from build123d import *

# Parameters (mm, degrees)
SALIENTE_EXTRUIR1_DEPTH = 2.5
CROQUIS2_R              = 3.175
CORTAR_EXTRUIR1_DEPTH   = 86.532786696


with BuildPart() as part:
    # Croquis1 → Saliente-Extruir1 (new, symmetric)
    with BuildSketch(Plane.XY):
        with BuildLine():
            Line((-85.24, 5), (85.24, 5))
            Line((85.24, 5), (85.24, -1))
            ThreePointArc((85.24, -1), (84.068427125, -3.828427125), (81.24, -5))
            Line((81.24, -5), (-81.24, -5))
            ThreePointArc((-81.24, -5), (-84.068427125, -3.828427125), (-85.24, -1))
            Line((-85.24, -1), (-85.24, 5))
        make_face()
    extrude(amount=SALIENTE_EXTRUIR1_DEPTH, both=True)

    # Croquis2 → Cortar-Extruir1 (cut, through all)
    with BuildSketch(Plane.XY.offset(2.5)):
        with Locations((42.62, 0)):
            Circle(CROQUIS2_R)
        with Locations((-42.62, 0)):
            Circle(CROQUIS2_R)
    extrude(amount=-CORTAR_EXTRUIR1_DEPTH, mode=Mode.SUBTRACT)


solid = part.part
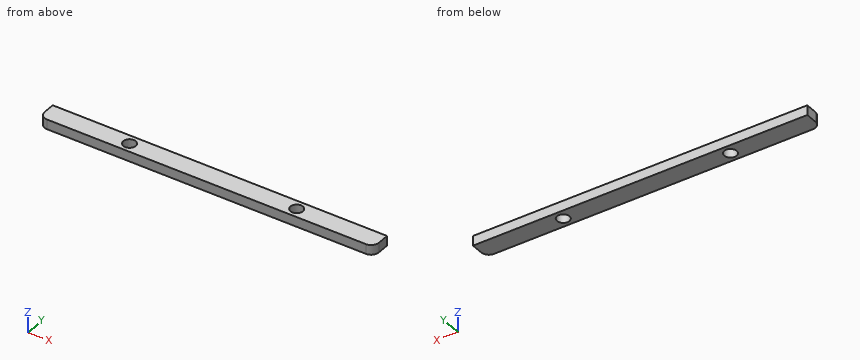
Geometry check sheet. Reference: the model listing, model coordinates, mm. Give positions to 0.01 mm unless a question says otherwise; leave off trailing zeros. Write each loop counter-clockwise with the first axis right and the second up, starting at its lowest first coordinate (ties: lowest second). Pieces come first, ordered by that corner, then holes. Notation, with made-up numbers: M 36,54.5 L 47,54.5 A7 cw 47,60.5 Z; hole C 9,18 d5. An arc over 180 degrees is marked long. Answer as CSV lines item,"result". Start each with the question number.
Q1. Material ranges on L1, parallel to Y at x = -42.62, z = 0.25 (3 decimals); L2, parallel to X at y = 2.25, z = 1.05; L3, parallel to X at y = 1.5, z = -1.9, recorded low to high.
Q2. Section check C-C, the plane y = 1.5. Record the cut outline in (x, z).
Q3. Section check A-A, the plane x = -42.62. Record the cut outline in (y, z) (3 decimals).
Q4. Section check B-B, the plane z = 0.6. Record the cut outline in (x, y) (3 decimals), then the cut area to 3 significant figures.
Geometry says:
1,L1,"-5 to -3.175, 3.175 to 5"
1,L2,"-85.24 to -44.86, -40.38 to 40.38, 44.86 to 85.24"
1,L3,"-85.24 to -45.42, -39.82 to 39.82, 45.42 to 85.24"
2,outline,"M -85.24,-2.5 L -45.42,-2.5 L -45.42,2.5 L -85.24,2.5 Z; M -39.82,-2.5 L 39.82,-2.5 L 39.82,2.5 L -39.82,2.5 Z; M 45.42,-2.5 L 85.24,-2.5 L 85.24,2.5 L 45.42,2.5 Z"
3,outline,"M -5,-2.5 L -3.175,-2.5 L -3.175,2.5 L -5,2.5 Z; M 3.175,-2.5 L 5,-2.5 L 5,2.5 L 3.175,2.5 Z"
4,outline,"M -85.24,-1 A4 ccw -81.24,-5 L 81.24,-5 A4 ccw 85.24,-1 L 85.24,5 L -85.24,5 Z; hole C -42.62,0 d6.35; hole C 42.62,0 d6.35"
4,area,"1,630 mm^2"
